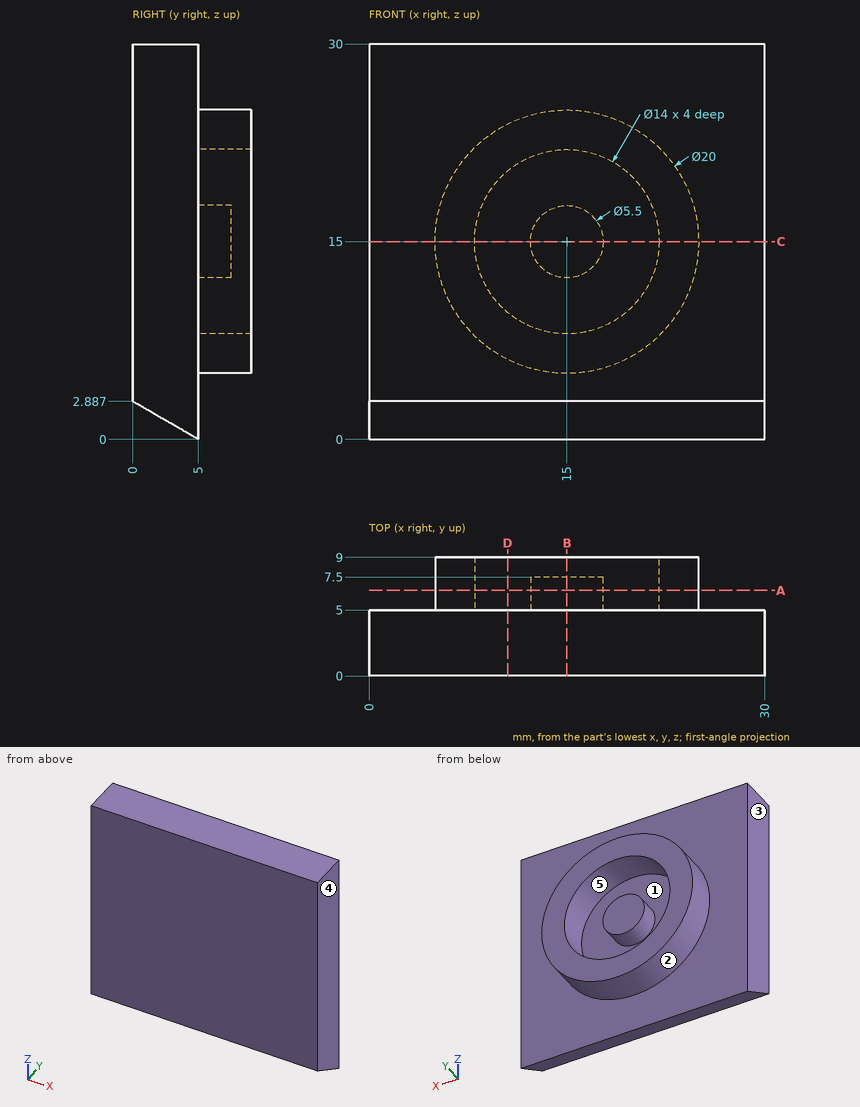
Geometry: see drawing. Coordinates: mm, zero at the bounding-box minimum. A direction names the side the tool comes from. Give positions to 0.01 mm unless a question says otherwise; leave off trailing zeros. Order: outer loops, then holes, each group sorted by start corner. A loop starts at its lowest first (then second) coordinate and runs counter-clockwise, first axis right, second up. Notation, with made-up numbers: (54.5, 85) -> (69.5, 85) arc R22 ccw to (69.5, 98) -> close; hole circle Ø4 at (-13, 47). An arc over 180 degrees is marked (long way). Write item = value, one per line.
Q1. Cut plane D-D, the plane x = 10.5. Output: boundary loops of the cut face in (y, z), and give its area (3 significant figures).
Data:
outline = (0, 2.89) -> (5, 0) -> (5, 6.07) -> (9, 6.07) -> (9, 9.64) -> (5, 9.64) -> (5, 20.36) -> (9, 20.36) -> (9, 23.93) -> (5, 23.93) -> (5, 30) -> (0, 30) -> close
area = 171 mm^2
Q2. Pin query (flat end, axial travel): pin 1 (3 mm diameter, centred on x = 7.5, y = 7.5, fed in from +Z); pin 2 (11 mm diameter, centred on x = 15, z = 13, fed in from +Y); pin 3 (1 mm diameter, centred on y = 7.5, z = 11.5, fed in from +X); pin 4 (4.5 mm diameter, centred on x = 16, z = 14, fed in from +Y). Return the tip coordinate at first contact, or that it passes through.
Data:
pin_1 = 23
pin_2 = 9
pin_3 = 24.54
pin_4 = 7.5
Q3. Pull-direction query (Z, two-part tool) for the marked faces 1, 2 and 3; classes: released by +Z, released by -Z, zero draft, split by the parting line, or undercut.
Data:
face_1 = undercut
face_2 = split by the parting line
face_3 = zero draft
Q4. Cut plane B-B, the plane x = 15. Output: boundary loops of the cut face in (y, z).
Data:
outline = (0, 2.89) -> (5, 0) -> (5, 5) -> (9, 5) -> (9, 8) -> (5, 8) -> (5, 12.25) -> (7.5, 12.25) -> (7.5, 17.75) -> (5, 17.75) -> (5, 22) -> (9, 22) -> (9, 25) -> (5, 25) -> (5, 30) -> (0, 30) -> close
Q5. Cut plane A-A, the plane y = 6.5. Output: boundary loops of the cut face in (x, z).
Data:
outline = circle Ø20 at (15, 15); circle Ø5.5 at (15, 15); hole circle Ø14 at (15, 15)
Q6. Set-up query: the marked faces 4 and 5. Return all of +Z, -Z, +X, -X, +Y, -Y with unobstructed straight access to the full face (end or side cutting, diameter ignored); none if empty.
Data:
face_4 = +Z, -Z, +X, +Y, -Y
face_5 = +Y
Q7. Material intervals for line 1 (Z direction, x = 15, y = 5.9); line 2 (Z direction, x = 16, y = 6.5); line 3 (X direction, y = 8.1, z = 15), sorted ascending. Write a range as from..to.
Data:
line_1 = 5..8, 12.25..17.75, 22..25
line_2 = 5.05..8.07, 12.44..17.56, 21.93..24.95
line_3 = 5..8, 22..25
Q8. Cut plane C-C, the plane z = 15. Output: boundary loops of the cut face in (x, y), and give its area (3 significant figures).
Data:
outline = (0, 0) -> (30, 0) -> (30, 5) -> (25, 5) -> (25, 9) -> (22, 9) -> (22, 5) -> (17.75, 5) -> (17.75, 7.5) -> (12.25, 7.5) -> (12.25, 5) -> (8, 5) -> (8, 9) -> (5, 9) -> (5, 5) -> (0, 5) -> close
area = 188 mm^2
